The listing builds one solid part. Answer for the finished solid, in the listing's coordinates (mm). Face numbers are marked on the shaded views. A direction names the side the tool comes from. Give positions to 0.01 mm unless a question says otherwise; leave off trailing zeros. Order: outer loops, then holes, each group sorted by start corner. A loop starts at its lowest first (then second) coordinate and runs counter-clockwise, first axis right, second up. Notation, with made-up numbers: (22.5, -23.5) - (30.5, -23.5) arc R22 ccw to (30.5, -16.5) - close; hole circle Ø3 at (-35.75, -39). An arc over 180 degrees is marked (long way). Answer as a JSON object with one key per item and string values. Group by question number.
Q1. For the marked faces 4, 5 and 6, determine the directions among +Z, -Z, +X, -X, +Y, -Y from which every point of the face is accessible in a straight line to the end or side of a thin tool.
Q2. A cutting plane is placed at A-A, the plane z = 45. Give the vertices of the cut face in (x, y).
Q3. Consider line 1 (Y direction, x = 78.75, z = 29.5); line 2 (X direction, y = 37.5, z = 26.5); line 3 (Z direction, x = 75, y = 53). Determine where each line is inside the solid, lowest interval first.
Q4. A cutting plane is placed at C-C, the plane z = 60.5. Give the vertices of the cut face in (x, y).
Q5. A cutting plane is placed at B-B, the plane x = 55. Give the vertices of the cut face in (y, z), and give its area (3 significant figures).
Q6. A cutting plane is placed at D-D, the plane y = 9. Give the vertices of the cut face in (x, z), and give its area (3 significant figures).
Q7. The mould has two halves that part along Y. Classify the marked faces 1, 2 and 3: released by +Y, released by -Y, zero draft, split by the parting line, or undercut.
Q8. Given pin 1 (3 mm diameter, centred on y = 36.59, z = 17.4, fed in from -X); pin 2 (6.5 mm diameter, centred on x = 18, z = 20.5, fed in from -Y); pin 3 (1.5 mm diameter, centred on y = 20, z = 49.5, fed in from -X); pin 4 (4 mm diameter, centred on y = 36.59, z = 17.4, fed in from +X), each flat-ended and moving along its own axis, determine where each tip first touches the part or whether it passes through.
Autodesk Inventor part; units mm, degrees
ref_plane "YZ Plane" through (0, 0, 0) normal (1, 0, 0) x (0, 1, 0)
ref_plane "XZ Plane" through (0, 0, 0) normal (0, 1, 0) x (-1, 0, 0)
ref_plane "XY Plane" through (0, 0, 0) normal (0, 0, 1) x (1, 0, 0)
sketch "Szkic1" plane through (0, 0, 0) normal (0, 0, 1) x (1, 0, 0)
  line L0 (0, 0) -> (120, 0)
  line L1 (0, 0) -> (10.4189, 59.0885)
  line L2 (0, 0) -> (60, 0) construction
  line L3 (120, 0) -> (97.4189, 29.0885)
  line L4 (10.4189, 59.0885) -> (70.4189, 59.0885)
  line L5 (10.4189, 59.0885) -> (70.4189, 59.0885) construction
  line L6 (97.4189, 29.0885) -> (97.4189, 59.0885)
  line L7 (97.4189, 59.0885) -> (70.4189, 59.0885)
  line L8 (20.4189, 49.0885) -> (70.4189, 49.0885)
  line L9 (70.4189, 49.0885) -> (70.4189, 24.0885)
  line L10 (70.4189, 24.0885) -> (20.4189, 24.0885)
  line L11 (20.4189, 24.0885) -> (20.4189, 49.0885)
  line L12 (20.4189, 49.0885) -> (14.4189, 49.0885)
  line L13 (14.4189, 49.0885) -> (14.4189, 24.0885)
  line L14 (14.4189, 24.0885) -> (20.4189, 24.0885)
  line L15 (20.4189, 24.0885) -> (20.4189, 49.0885)
  line L16 (70.4189, 49.0885) -> (80.4189, 49.0885)
  line L17 (80.4189, 49.0885) -> (80.4189, 24.0885)
  line L18 (80.4189, 24.0885) -> (70.4189, 24.0885)
  line L19 (70.4189, 24.0885) -> (70.4189, 49.0885)
  dimension "d0" = 120
  dimension "d1" = 60
  dimension "d2" = 80
  dimension "d4" = 60
  dimension "d5" = 0
  dimension "d6" = 50
  dimension "d7" = 25
  dimension "d8" = 10
  dimension "d9" = 10
  dimension "d10" = 6
  dimension "d11" = 10
  dimension "d23" = 27
  dimension "d24" = 30
extrude "Wyciągnięcie proste1" add sketch "Szkic1" along normal blind 5
extrude "Wyciągnięcie proste2" add sketch "Szkic1" along normal blind 30 contours L11 L14 L13 L12
extrude "Wyciągnięcie proste3" add sketch "Szkic1" along normal blind 50 contours L16 L17 L18 L9
sketch "Szkic2" plane through (70.4189, 49.0885, 5) normal (0, 1, 0) x (1, 0, 0)
  point P0 (-70.4189, 5)
sketch "Szkic3" plane through (70.4189, 49.0885, 5) normal (0, 1, 0) x (1, 0, 0)
  line L0 (0, 0) -> (0, -45)
  line L1 (-70.4189, 0) -> (49.5811, 0)
  line L2 (0, -45) -> (10, -45)
  line L3 (10, -45) -> (10, 0)
  line L4 (10, 0) -> (0, 0)
  line L5 (0, 0) -> (0, -45)
  point P0 (-70.4189, 5)
  dimension "d18" = 10
extrude "Wyciągnięcie proste4" add sketch "Szkic3" along normal blind 10
sketch "Szkic4" plane through (70.4189, 24.0885, 5) normal (0, -1, 0) x (1, 0, 0)
  line L0 (0, 45) -> (10, 45)
  line L1 (0, 0) -> (0, -5)
  line L2 (10, 45) -> (0, 45)
  line L3 (0, 45) -> (0, 0)
  line L4 (0, 0) -> (10, 0)
  line L5 (10, 0) -> (10, 45)
  point P0 (-70.4189, -5)
extrude "Wyciągnięcie proste5" add sketch "Szkic4" along normal up to surface (24.0885 mm away)
sketch "Szkic5" plane through (0, 0, 50) normal (0, 0, 1) x (1, 0, 0)
  line L0 (70.4189, 49.0885) -> (70.4189, 59.0885)
  line L1 (80.4189, 59.0885) -> (80.4189, 0)
  line L2 (70.4189, 59.0885) -> (80.4189, 59.0885)
  line L3 (80.4189, 59.0885) -> (80.4189, 0)
  line L4 (80.4189, 0) -> (70.4189, 0)
  line L5 (70.4189, 0) -> (70.4189, 59.0885)
  point P0 (0, 0)
extrude "Wyciągnięcie proste6" add sketch "Szkic5" along normal blind 20
sketch "Szkic6" plane through (70.4189, 24.0885, 0) normal (-1, 0, 0) x (0, 0, 1)
  line L0 (5, 35) -> (70, 35)
  line L1 (30, 25) -> (30, 0)
  point P0 (0, -24.0885)
  point P1 (45, 12.5)
  point P2 (30, 12.5)
  dimension "d27" = 22.5
  dimension "d28" = 15
hole "Otwór1" at (70.4189, 36.5885, 45) direction (1, 0, 0) diameter 7 end through all
sketch "Szkic7" plane through (80.4189, 0, 5) normal (1, 0, 0) x (0, 0, -1)
  line L0 (0, 59.0885) -> (-65, 59.0885)
  line L1 (0, 0) -> (0, 24.0885)
  line L2 (-65, 59.0885) -> (0, 59.0885)
  line L3 (0, 59.0885) -> (0, 0)
  line L4 (0, 0) -> (-65, 0)
  line L5 (-65, 0) -> (-65, 59.0885)
  circle A0 centre (-40, 36.5885) radius 3.5
  circle A1 centre (-40, 36.5885) radius 3.5
  point P0 (5, 0)
extrude "Wyciągnięcie proste7" add sketch "Szkic7" along normal blind 2
sketch "Szkic8" plane through (70.4189, 24.0885, 0) normal (-1, 0, 0) x (0, 0, 1)
  line L0 (5, 35) -> (70, 35)
  line L1 (5, -24.0885) -> (70, -24.0885)
  line L2 (5, 35) -> (70, 35)
  line L3 (70, 35) -> (70, -24.0885)
  line L4 (70, -24.0885) -> (5, -24.0885)
  line L5 (5, -24.0885) -> (5, 35)
  line L6 (5, 35) -> (70, 35)
  line L7 (70, 35) -> (70, -24.0885)
  line L8 (70, -24.0885) -> (5, -24.0885)
  line L9 (5, -24.0885) -> (5, 35)
  circle A0 centre (45, 12.5) radius 3.5
  circle A1 centre (45, 12.5) radius 3.5
  point P0 (0, -24.0885)
  point P1 (70, 35)
extrude "Wyciągnięcie proste8" cut sketch "Szkic8" against normal blind 2
sketch "Szkic9" plane through (82.4189, 0, 5) normal (1, 0, 0) x (0, 0, -1)
  circle A0 centre (-40, 36.5885) radius 3.5
  point P0 (5, 0)
  point P1 (-55.5, 52.0885)
  point P2 (-24.5, 52.0885)
  point P3 (-24.5, 52.0885)
  point P4 (-24.5, 21.0885)
  point P5 (-55.5, 21.0885)
  dimension "d40" = 31
  dimension "d41" = 31
  dimension "d42" = 31
  dimension "d43" = 31
  dimension "d44" = 15.5
  dimension "d45" = 15.5
hole "Otwór2" at (82.4189, 52.0885, 60.5) at (82.4189, 52.0885, 29.5) at (82.4189, 21.0885, 60.5) at (82.4189, 21.0885, 29.5) direction (-1, 0, 0) diameter 3.4 end through all
sketch "Szkic10" plane through (14.4189, 24.0885, 5) normal (-1, 0, 0) x (0, 0, 1)
  point P0 (-5, -24.0885)
  point P1 (12.3965, 12.5)
hole "Otwór3" at (14.4189, 36.5885, 17.3965) direction (1, 0, 0) diameter 3.4 end through all
sketch "Szkic12" plane through (0, 0, 5) normal (0, 0, 1) x (1, 0, 0)
  line L0 (20.4189, 49.0885) -> (70.4189, 49.0885)
  line L1 (70.4189, 49.0885) -> (70.4189, 54.0885)
  line L2 (70.4189, 54.0885) -> (45.4189, 54.0885)
  line L3 (70.4189, 24.0885) -> (20.4189, 24.0885)
  line L4 (70.4189, 24.0885) -> (70.4189, 19.0885)
  line L5 (70.4189, 19.0885) -> (45.4189, 19.0885)
  line L6 (45.4189, 19.0885) -> (45.4189, 54.0885)
  point P0 (0, 0)
  point P1 (45.4189, 24.0885)
  point P2 (45.4189, 49.0885)
  dimension "d63" = 5
  dimension "d64" = 5
extrude "Wyciągnięcie proste10" cut sketch "Szkic12" against normal blind 10
properties part number "podstawka pod silnik"
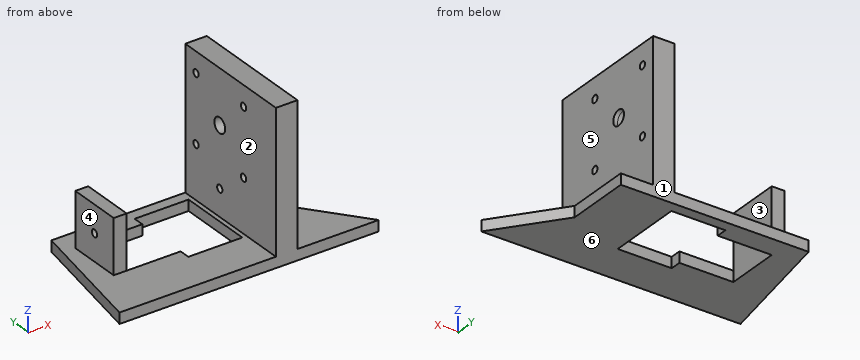
Reply:
{
 "1": {"face 4": "+Z, -X, +Y, -Y", "face 5": "+Z, +X, +Y, -Y", "face 6": "-Z, +X, -X, +Y, -Y"},
 "2": {"outline": "(72.42, 0) - (82.42, 0) - (82.42, 33.09) - (72.42, 33.09) - close; (72.42, 40.09) - (82.42, 40.09) - (82.42, 59.09) - (72.42, 59.09) - close"},
 "3": {"line 1": "y = 0 to 19.39, 22.79 to 50.39, 53.79 to 59.09", "line 2": "x = 14.42 to 20.42, 72.42 to 82.42", "line 3": "z = 0 to 28.07, 30.93 to 59.07, 61.93 to 70"},
 "4": {"outline": "(72.42, 0) - (82.42, 0) - (82.42, 19.39) - (72.42, 19.39) - close; (72.42, 22.79) - (82.42, 22.79) - (82.42, 50.39) - (72.42, 50.39) - close; (72.42, 53.79) - (82.42, 53.79) - (82.42, 59.09) - (72.42, 59.09) - close"},
 "5": {"outline": "(0, 0) - (19.09, 0) - (19.09, 5) - (0, 5) - close; (54.09, 0) - (59.09, 0) - (59.09, 5) - (54.09, 5) - close", "area": "120 mm^2"},
 "6": {"outline": "(1.59, 0) - (113.01, 0) - (113.01, 5) - (82.42, 5) - (82.42, 70) - (72.42, 70) - (72.42, 5) - (1.59, 5) - close", "area": "1,210 mm^2"},
 "7": {"face 1": "released by +Y", "face 2": "zero draft", "face 3": "undercut"},
 "8": {"pin 1": "passes through", "pin 2": "stops at y = 24.09", "pin 3": "stops at x = 72.42", "pin 4": "stops at x = 82.42"}
}
